Autodesk Inventor part; units mm, degrees
ref_plane "YZ Plane" through (0, 0, 0) normal (1, 0, 0) x (0, 1, 0)
ref_plane "XZ Plane" through (0, 0, 0) normal (0, 1, 0) x (-1, 0, 0)
ref_plane "XY Plane" through (0, 0, 0) normal (0, 0, 1) x (1, 0, 0)
sketch "Sketch1" plane through (0, 0, 0) normal (0, 0, 1) x (1, 0, 0)
  line L0 (0, 0) -> (-8, 0)
  line L1 (-8, 0) -> (-8, 50)
  line L2 (-8, 50) -> (0, 50)
  line L3 (0, 50) -> (0, 0)
  circle A0 centre (-4, 38) radius 1.6
  circle A1 centre (-4, 12) radius 1.6
  line L4 (0, 34) -> (6.1, 34)
  line L5 (6.1, 34) -> (6.1, 16)
  line L6 (6.1, 16) -> (0, 16)
  line L7 (0, 16) -> (0, 34)
  point P0 (-4, 50)
  point P1 (-4, 0)
  point P2 (0, 25)
  dimension "d0" = 8
  dimension "d1" = 50
  dimension "d2" = 3.2
  dimension "d3" = 3.2
  dimension "d18" = 6.1
  dimension "d19" = 18
  dimension "d28" = 4
  dimension "d29" = 4
extrude "Extrusion1" add sketch "Sketch1" along normal blind 5
sketch "Sketch2" plane through (0, 0, 5) normal (0, 0, 1) x (1, 0, 0)
  line L0 (-8, 0) -> (0, 0)
  line L1 (0, 50) -> (-8, 50)
  line L2 (-8, 50) -> (0, 50)
  line L3 (0, 50) -> (0, 42)
  line L4 (0, 42) -> (-8, 42)
  line L5 (-8, 42) -> (-8, 50)
  line L6 (-8, 0) -> (0, 0)
  line L7 (0, 0) -> (0, 8)
  line L8 (0, 8) -> (-8, 8)
  line L9 (-8, 8) -> (-8, 0)
  dimension "d8" = 8
  dimension "d10" = 8
extrude "Extrusion2" add sketch "Sketch2" along normal blind 14.4
sketch "Sketch3" plane through (0, 0, 0) normal (1, 0, 0) x (0, 0, -1)
  circle A0 centre (-16.4, 46) radius 1.6
  circle A1 centre (-16.4, 4) radius 1.6
  line L0 (-19.4, 42) -> (-19.4, 50)
  line L1 (-19.4, 0) -> (-19.4, 8)
  point P0 (0, 0)
  point P1 (-19.4, 46)
  point P2 (-19.4, 4)
  dimension "d13" = 3.2
  dimension "d14" = 3.2
  dimension "d15" = 3
extrude "Extrusion3" cut sketch "Sketch3" against normal blind 15
sketch "Sketch4" plane through (0, 0, 5) normal (0, 0, 1) x (1, 0, 0)
  line L0 (6.1, 16) -> (6.1, 34)
  line L1 (6.1, 34) -> (2.1, 34)
  line L2 (2.1, 34) -> (2.1, 16)
  line L3 (2.1, 16) -> (6.1, 16)
  line L4 (6.1, 16) -> (6.1, 34)
  line L5 (0, 16) -> (6.1, 16)
  line L6 (6.1, 34) -> (0, 34) construction
  line L7 (-4, 34) -> (0, 34)
  line L8 (0, 34) -> (0, 16)
  line L9 (0, 16) -> (-4, 16)
  line L10 (-4, 16) -> (-4, 34)
  point P0 (0, 0)
  dimension "d21" = 4
  dimension "d26" = 4
  dimension "d27" = 2.1
extrude "Extrusion4" add sketch "Sketch4" along normal blind 8
equation "\"d29\" = d28"
equation "\"d8\" = d10"
properties part number "X rollers"
Source: CAD feature listing. Evaluate the final solid. Frame: model axes, mm. A direction names the side the tool comes from. Round coordinates to 2 decimals unless told otherwise and drop trailing zeros. Write each loop counter-clockwise with the first axis right and the second up, starting at its lowest first coordinate (ties: lowest second). Pieces come first, ordered by that corner, then holes. Notation, with made-up numbers: M -40,9 L -5,9 A23 ccw -5,27 Z; hole C 89.25,64 d11. An arc over 180 degrees is marked long. Use CSV: the item, a comma, the result in double quotes. Start each with the question number.
Q1. Pull-direction query (X, two-part tool) for faces 1 (the face through (-2, 25, 13)), 2 (the face through (0, 25, 9)), 3 (the face through (0, 6, 7)), 4 (the face through (2.1, 25, 9)); classes: +X half, -X half, draft (parallel to the pull), parting line (faces both ways), or undercut.
Q2. Access query for faces 5 (the face through (-2, 16, 9)), 6 (the face through (1, 25, 5)), 7 (the face through (-3.94, 44.58, 15.66)), 8 (the face through (4, 25, 13)), 9 (the face through (4, 34, 6)). Directions: +Z, -Z, +X, -X, +Y, -Y. A direction counts if a zero-diameter tool reaches every point of the face in a straight line with its end or side. Return the directions, or none.
Q3. First-contact query: P1, Ø1.8, axis at x = 2, z = 8, coming from the +Y side; P2, Ø1.2, axis at x = -1.5, y = 27, coming from the +Z side; P3, Ø5, axis at x = 4, z = 8, coming from the -Y side. Flat tips, straight axial feed; report the tip coordinate or a pass-through.
Q4. Cut plane C-C on z = 16.4. Output: boundary loops of the cut face in (x, y).
Q5. Line query: line 1 (Y direction, x = -6.5, z = 16.4); line 2 (Y direction, x = -1, z = 7); line 3 (Y direction, x = -1.5, z = 16). Output: solid intervals per line, ascending. Write a range as from..to.
Q6. Cut plane B-B on z = 13.5. Output: boundary loops of the cut face in (x, y).
Q7. Cut plane D-D on x = -6.25. Output: boundary loops of the cut face in (y, z), plus the area to 3 significant figures.
Q8. Cut plane A-A on y = 38. Output: boundary loops of the cut face in (x, z), plus the area to 3 significant figures.
Results found:
1,face 1,"draft"
1,face 2,"undercut"
1,face 3,"+X half"
1,face 4,"undercut"
2,face 5,"+Z, +X, -X"
2,face 6,"+Z, +Y, -Y"
2,face 7,"+X, -X"
2,face 8,"+Z, +X, -X, +Y, -Y"
2,face 9,"+Z, -Z, +X, +Y"
3,P1,"y = 34"
3,P2,"z = 13"
3,P3,"y = 16"
4,outline,"M -8,0 L 0,0 L 0,2.4 L -8,2.4 Z; M -8,5.6 L 0,5.6 L 0,8 L -8,8 Z; M -8,42 L 0,42 L 0,44.4 L -8,44.4 Z; M -8,47.6 L 0,47.6 L 0,50 L -8,50 Z"
5,line 1,"0..2.4, 5.6..8, 42..44.4, 47.6..50"
5,line 2,"0..8, 16..34, 42..50"
5,line 3,"0..2.45, 5.55..8, 42..44.45, 47.55..50"
6,outline,"M -8,0 L 0,0 L 0,8 L -8,8 Z; M -8,42 L 0,42 L 0,50 L -8,50 Z"
7,outline,"M 0,0 L 50,0 L 50,19.4 L 42,19.4 L 42,5 L 8,5 L 8,19.4 L 0,19.4 Z; hole C 4,16.4 d3.2; hole C 46,16.4 d3.2"
7,area,"464 mm^2"
8,outline,"M -8,0 L -5.6,0 L -5.6,5 L -8,5 Z; M -2.4,0 L 0,0 L 0,5 L -2.4,5 Z"
8,area,"24.0 mm^2"
